Work out the finished part from the listing and answer in its coordinate system (mm). Coordinates: 2 decimals unless noted, no trailing zeros. Order: outer loops, then holes, each group sorted by start corner. A loop starts at its lowest first (then second) coordinate and runs counter-clockwise, first axis right, second up. Notation, with made-up numbers: M -12,-10 L 11,-10 A21 ccw 11,17 Z; hole C -32,70.5 d8. An arc over 180 degrees is marked long. Write item = value, one per line. Start each with the question number.
Q1. Straight lines are drawn through the part: line 1 along X through (y, z) = (164.5, 1.2); line 2 along Y through (x, z) = (-187, 0.65); line 3 along X through (y, z) = (120.5, 0.15). For each, find the intervals that lie inside material, in ascending order.
Q2. Each of these flat-tipped pins is pushed along its axis until it touches: P1, Ø1, axis at y = 183.5, z = 0.5, coming from the -X side; P2, Ø1, axis at y = 158, z = 1, coming from the -X side; P3, Ø1, axis at x = -227, z = 1, coming from the +Y side. Where does it stop, or does it pass through?
Q3. Find section A-A on y = 96. Give the vertices of the cut face in (x, z), and give its area (3 significant figures).
Q4. Find section B-B on z = 1.45. Give the number of separate pieces and of enclosed holes in the cut face, and give its area (3 significant figures).
```python
from build123d import *

# Parameters (mm, degrees)
SKETCH_1_R      = 1.52
EXTRUDE_1_DEPTH = 2


with BuildPart() as part:
    # 草图1 → 凸台-拉伸1 (new body)
    with BuildSketch(Plane.XY):
        Polygon((-122.332772904, 193.928670444), (-130.112569709, 209.893801205), (-139.698830821, 214.194588314), (-145.581311392, 201.082803585), (-172.906818534, 173.07089056), (-181.550834018, 175.272509679), (-192.956593094, 163.580242467), (-190.541243439, 154.993495907), (-211.394103482, 133.616820304), (-220.038118966, 135.818439423), (-231.443878041, 124.126172211), (-229.028528386, 115.539425652), (-256.354035527, 87.527512628), (-269.315875894, 81.321614566), (-264.778632454, 71.844980469), (-248.625442054, 64.46357962), (-240.711857184, 72.575950598), (-244.144105033, 81.654022148), (-219.836292658, 106.572437113), (-211.192277174, 104.370817994), (-199.786518099, 116.063085206), (-202.201867754, 124.649831766), (-181.34900771, 146.026507369), (-172.704992227, 143.82488825), (-161.299233151, 155.517155462), (-163.714582806, 164.103902021), (-139.406770431, 189.022316987), (-130.246357773, 185.816299466), align=None)
        with Locations((-259.604526823, 80.250654079)):
            Circle(SKETCH_1_R, mode=Mode.SUBTRACT)
        with Locations((-251.678290532, 76.597666862)):
            Circle(SKETCH_1_R, mode=Mode.SUBTRACT)
        with Locations((-234.858840543, 100.367593581)):
            Circle(SKETCH_1_R, mode=Mode.SUBTRACT)
        with Locations((-221.201454913, 114.368047313)):
            Circle(SKETCH_1_R, mode=Mode.SUBTRACT)
        with Locations((-221.341779466, 125.680885552)):
            Circle(SKETCH_1_R, mode=Mode.SUBTRACT)
        with Locations((-210.028941227, 125.821210105)):
            Circle(SKETCH_1_R, mode=Mode.SUBTRACT)
        with Locations((-196.371555596, 139.821663837)):
            Circle(SKETCH_1_R, mode=Mode.SUBTRACT)
        with Locations((-182.714169966, 153.822117568)):
            Circle(SKETCH_1_R, mode=Mode.SUBTRACT)
        with Locations((-171.401331727, 153.962442121)):
            Circle(SKETCH_1_R, mode=Mode.SUBTRACT)
        with Locations((-182.854494518, 165.134955807)):
            Circle(SKETCH_1_R, mode=Mode.SUBTRACT)
        with Locations((-171.541656279, 165.27528036)):
            Circle(SKETCH_1_R, mode=Mode.SUBTRACT)
        with Locations((-157.884270649, 179.275734092)):
            Circle(SKETCH_1_R, mode=Mode.SUBTRACT)
        with Locations((-134.538850305, 196.679603292)):
            Circle(SKETCH_1_R, mode=Mode.SUBTRACT)
        with Locations((-138.387317573, 204.512791471)):
            Circle(SKETCH_1_R, mode=Mode.SUBTRACT)
        with Locations((-209.888616674, 114.508371866)):
            Circle(SKETCH_1_R, mode=Mode.SUBTRACT)
    extrude(amount=EXTRUDE_1_DEPTH)


solid = part.part
```
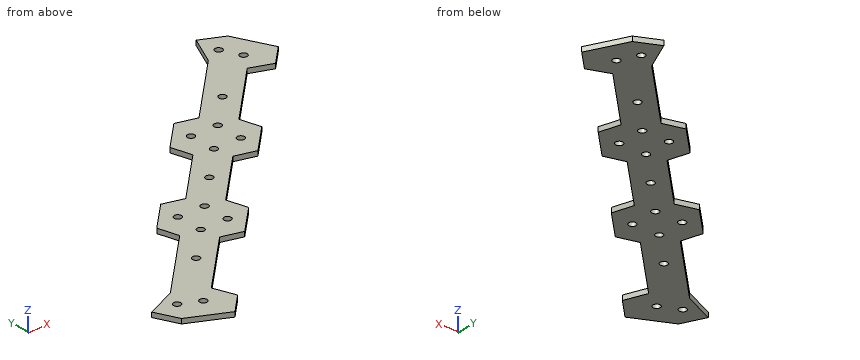
Findings below:
q1.line_1 = -192.06 to -184.24, -181.47 to -172.85, -170.23 to -163.33
q1.line_2 = 140.23 to 169.69
q1.line_3 = -230.42 to -201.03
q2.P1 = -163.22
q2.P2 = -191.53
q2.P3 = 129.19
q3.outline = M -248.09,0 L -230.15,0 L -230.15,2 L -248.09,2 Z
q3.area = 35.9 mm^2
q4.separate_pieces = 1
q4.enclosed_holes = 15
q4.area = 3,320 mm^2
